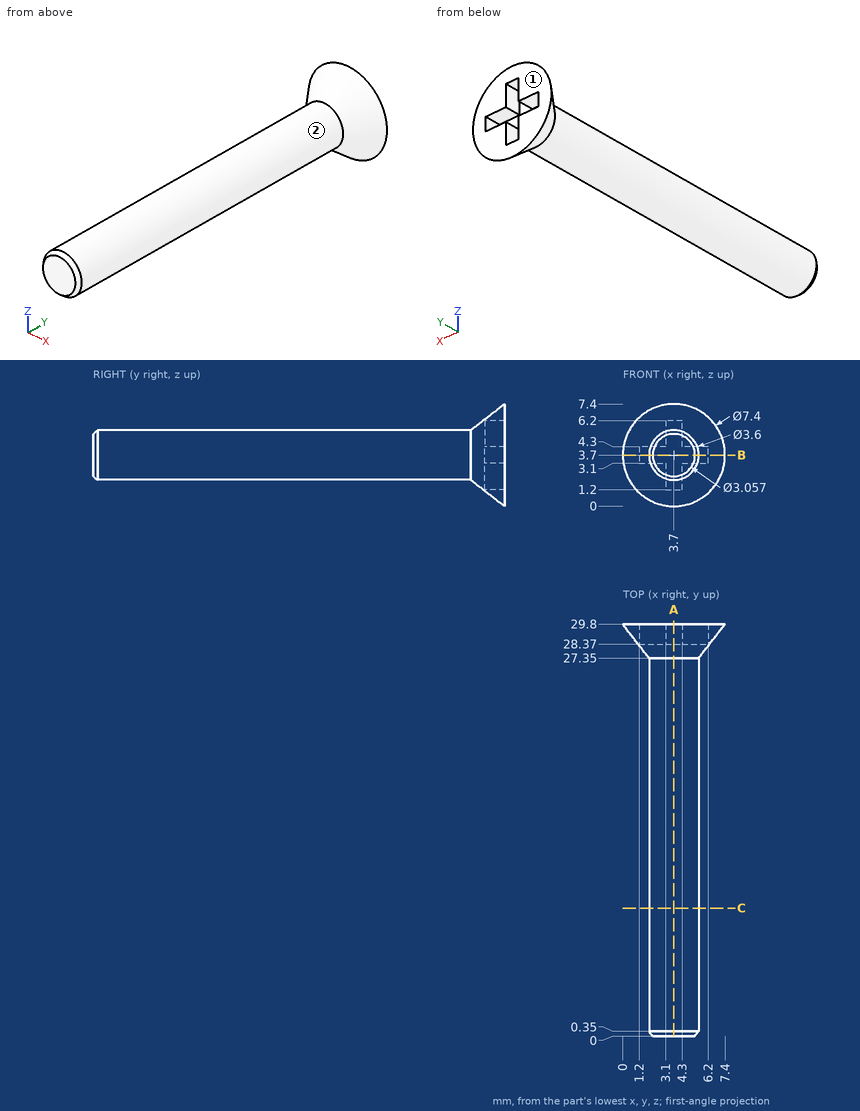
Could you check a few things on this drawing? It's one solid part, dimensions in mm from its lowest x, y, z. A direction names the side the tool comes from. Give positions to 0.01 mm unless a question says otherwise; leave off trailing zeros. Order: outer loops, then holes, each group sorted by start corner. A loop starts at its lowest first (then second) coordinate and runs counter-clockwise, first axis right, second up. Notation, with made-up numbers: (38, -12.75) - (57, -12.75) arc R26 cw to (57, 21.25) - close; hole circle Ø10 at (83, -5). An arc over 180 degrees is marked (long way). Answer as a JSON object with one key per item and string values. Group by question number.
Item 1: Which directions (+Z, -Z, +X, -X, +Y, -Y) give clear straight access to the entire face, cutting with the end or side of a thin tool? Please do the marked faces 1 and 2.
Item 2: For P1, Ø0.7, axis at x = 2.5, y = 29, coming from the -Z side (1 decimal); P2, Ø3, axis at y = 24.5, z = 4.5, coming from the -X side; P3, Ø1, axis at x = 3.5, y = 29, coming from the +Z side, each with a flat end and sliding along its axis, tell me the tip position at first contact or that it passes through.
Item 3: If we section it at A-A on x = 3.7: Please give me the cut outline in (y, z), and give its area (3 significant figures).
Item 4: If we section it at B-B on z = 3.7: Please give me the cut outline in (x, y), and give its area (3 significant figures).
Item 5: If we section it at C-C on y = 9.25: Please give me the cut outline in (x, z).
Item 6: Please list where these lines run through material, in increasing order: probe 1 along Y at (x, z) = (5, 3.75); probe 2 along X at (y, z) = (18, 3.75); probe 3 along Y at (x, z) = (6.5, 4.75) (1 decimal).
Result set:
{
 "1": {"face 1": "+Z, -Z, +X, -X, +Y", "face 2": "-Y"},
 "2": {"P1": "z = 0.5", "P2": "x = 1.9", "P3": "z = 7.16"},
 "3": {"outline": "(0, 2.17) - (0.35, 1.9) - (27.35, 1.9) - (29.8, 0) - (29.8, 1.2) - (28.37, 1.2) - (28.37, 6.2) - (29.8, 6.2) - (29.8, 7.4) - (27.35, 5.5) - (0.35, 5.5) - (0, 5.23) - close", "area": "105 mm²"},
 "4": {"outline": "(0, 29.8) - (1.9, 27.35) - (1.9, 0.35) - (2.17, 0) - (5.23, 0) - (5.5, 0.35) - (5.5, 27.35) - (7.4, 29.8) - (6.2, 29.8) - (6.2, 28.37) - (1.2, 28.37) - (1.2, 29.8) - close", "area": "105 mm²"},
 "5": {"outline": "circle Ø3.6 at (3.7, 3.7)"},
 "6": {"probe 1": "0 to 28.37", "probe 2": "1.9 to 5.5", "probe 3": "28.9 to 29.8"}
}
